Geometry check sheet. Reference: drawing and pictorial views, mm from the part's lowest x, y, z. A direction names the side the tool comes from. Give positions to 0.01 mm unless a question says otherwise; leave off trailing zeros. Order: outer loops, then holes, each group sorted by start corner. A loop starts at its lowest first (then second) coordinate and runs counter-clockwise, first axis right, second up. Notation, with made-up numbers: M 25,55 L 59,55 A28 ccw 59,77 Z; hole C 51,56.25 d9. An arc over 180 degrees is marked long. Answer as a JSON object with one key per item and string values. Group by question number.
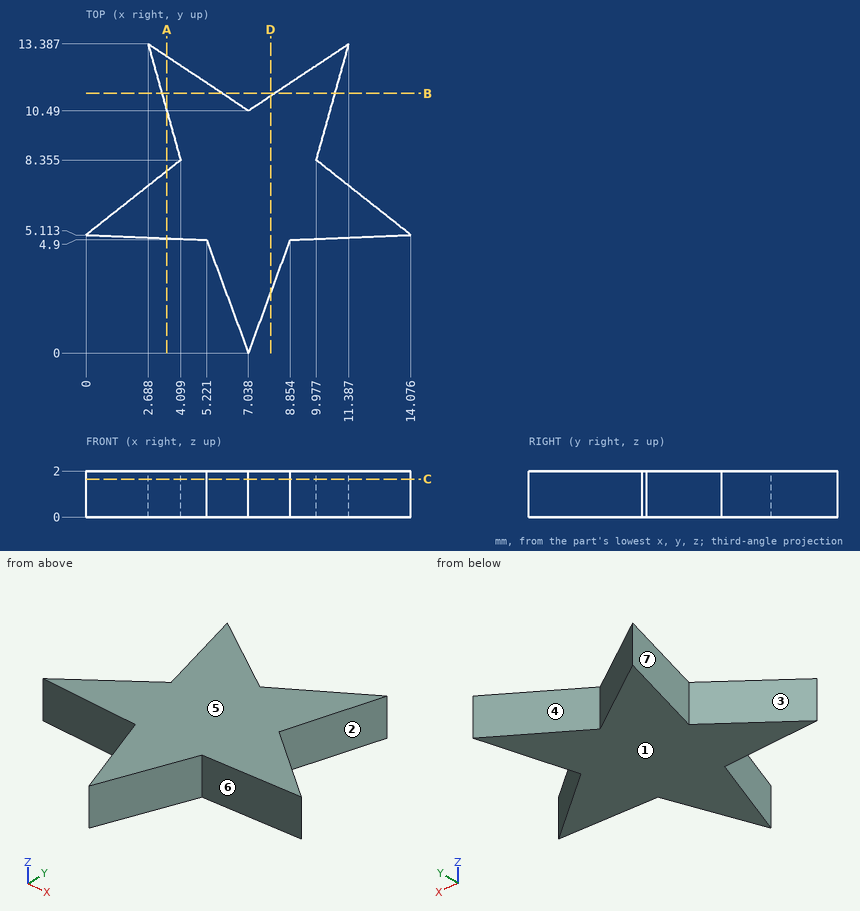
1. Cross-section at D-D (x = 8). Record the cut outline in (y, z) (1 decimal).
2. Thickness scan on line 1 along Y through (x, z) = (12.25, 1.4) (1 decimal); line 2 along Y through (x, z) = (5, 1.25); line 3 along X through (y, z) = (11.25, 1.8) (1 decimal). Record the ranges inside material, lowest first. Write a range as [from, to].
3. Cross-section at B-B (y = 11.25). Record the cut outline in (x, z).
4. Access from +Z, -Z, +X, -X, +Y, -Y to the whole of each face (thin tool, end or side, straight path). Record for the marked faces 1, 2, 3 and 4.
5. Cross-section at C-C (z = 1.65). Record the cut outline in (x, y) (1 decimal).
6. Release check for a two-part mould opening along Y. For the marked faces 5, 6 and 7 record: released by +Y, released by -Y, zero draft, split by the parting line, or undercut.
7. Cross-section at A-A (x = 3.5). Record the cut outline in (y, z).
Report:
{
 "1": {"outline": "M 2.6,0 L 11.1,0 L 11.1,2 L 2.6,2 Z"},
 "2": {"line 1": "y = [5, 6.6]", "line 2": "y = [4.91, 11.85]", "line 3": "x = [3.3, 5.9], [8.2, 10.8]"},
 "3": {"outline": "M 3.29,0 L 5.9,0 L 5.9,2 L 3.29,2 Z; M 8.18,0 L 10.79,0 L 10.79,2 L 8.18,2 Z"},
 "4": {"face 1": "-Z, +X, -X, +Y, -Y", "face 2": "+Z, -Z, +X", "face 3": "+Z, -Z, -X", "face 4": "+Z, -Z, +Y"},
 "5": {"outline": "M 0,5.1 L 5.2,4.9 L 7,0 L 8.9,4.9 L 14.1,5.1 L 10,8.4 L 11.4,13.4 L 7,10.5 L 2.7,13.4 L 4.1,8.4 Z"},
 "6": {"face 5": "zero draft", "face 6": "released by -Y", "face 7": "undercut"},
 "7": {"outline": "M 4.97,0 L 7.88,0 L 7.88,2 L 4.97,2 Z; M 10.49,0 L 12.85,0 L 12.85,2 L 10.49,2 Z"}
}
